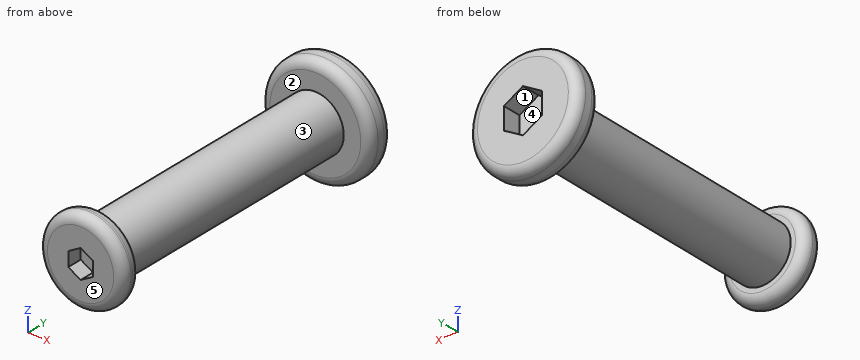
from build123d import *

# Parameters (mm, degrees)
SKETCH_1_R          = 2.9
EXTRUDE_1_DEPTH     = 1.4
CUT_EXTRUDE_1_DEPTH = 1
SKETCH_3_R          = 1.5
EXTRUDE_2_DEPTH     = 14
SKETCH_4_R          = 2.25
EXTRUDE_3_DEPTH     = 1.1
CUT_EXTRUDE_2_DEPTH = 0.8
FILLET_1_R          = 0.5


with BuildPart() as part:
    # 草图1 → 凸台-拉伸1 (new body)
    with BuildSketch(Plane(origin=(0, 0, 0), x_dir=(1, 0, 0), z_dir=(0, 1, 0))):
        with Locations(Location((0, 0, 0), (0, 0, 270))):
            Circle(SKETCH_1_R)
    extrude(amount=EXTRUDE_1_DEPTH)

    # 草图2 → 切除-拉伸1 (cut)
    with BuildSketch(Plane(origin=(0, 1.4, 0), x_dir=(1, 0, 0), z_dir=(0, 1, 0))):
        Polygon((1, 0.577350269), (0, 1.154700538), (-1, 0.577350269), (-1, -0.577350269), (0, -1.154700538), (1, -0.577350269), align=None)
    extrude(amount=-CUT_EXTRUDE_1_DEPTH, mode=Mode.SUBTRACT)

    # 草图3 → 凸台-拉伸2 (add)
    with BuildSketch(Plane.XZ):
        with Locations(Location((0, 0, 0), (0, 0, 270))):
            Circle(SKETCH_3_R)
    extrude(amount=EXTRUDE_2_DEPTH)

    # 草图4 → 凸台-拉伸3 (add)
    with BuildSketch(Plane.XZ.offset(14)):
        with Locations(Location((0, 0, 0), (0, 0, 270))):
            Circle(SKETCH_4_R)
    extrude(amount=EXTRUDE_3_DEPTH)

    # 草图5 → 切除-拉伸2 (cut)
    with BuildSketch(Plane.XZ.offset(15.1)):
        Polygon((0.65, 0.375277675), (0, 0.75055535), (-0.65, 0.375277675), (-0.65, -0.375277675), (0, -0.75055535), (0.65, -0.375277675), align=None)
    extrude(amount=-CUT_EXTRUDE_2_DEPTH, mode=Mode.SUBTRACT)

    # 圆角1
    fillet_1_edges = [part.edges().sort_by_distance(p)[0] for p in [
        (0, 0, -2.9),
        (0, -14, 2.25),
        (0, -15.1, 2.25),
        (0, 1.4, -2.9),
    ]]
    fillet(fillet_1_edges, radius=FILLET_1_R)


solid = part.part
Could you check a few things on this model? Use its own coordinates, in mm. Face numbers are marked on the shaded views. A direction names the side the tool comes from. Round coordinates to 2 decimals unless told otherwise and drop trailing zeros. Order: outer loops, then holes, each group sorted by start corner. A loop starts at its lowest first (then second) coordinate and runs counter-clockwise, first axis right, second up.
Q1. Imagine slicing it at B-B, the plane y = -3.25. List the corners of the cut face in (x, z) for me.
Geometry says:
outline: circle Ø3 at (0, 0)
Q2. I'm going to push flat-ended pins straight in: P1, Ø0.8, axis at y = -15, z = 0, coming from the +X side; P2, Ø0.7, axis at x = 0, z = 0, coming from the -Y side; P3, Ø1.5, axis at y = -8.5, z = 0, coming from the +X side. Where does each tip first touch, or does it pass through?
Geometry says:
P1: stops at x = 2.25
P2: stops at y = -14.3
P3: stops at x = 1.5
Q3. Which directions (+Z, -Z, +X, -X, +Y, -Y) give clear straight access to the entire face, cutting with the end or side of a thin tool? Please do the marked faces 4 and 5.
Geometry says:
face 4: +Y
face 5: +Z, -Z, +X, -X, -Y
Q4. Imagine slicing it at A-A, the plane z = 0. List the corners of the cut face in (x, y) for me, then the cut area to 3 significant figures.
Geometry says:
outline: (-2.9, 0.5) arc R0.5 ccw to (-2.4, 0) - (-1.5, 0) - (-1.5, -14) - (-1.75, -14) arc R0.5 ccw to (-2.25, -14.5) - (-2.25, -14.6) arc R0.5 ccw to (-1.75, -15.1) - (-0.65, -15.1) - (-0.65, -14.3) - (0.65, -14.3) - (0.65, -15.1) - (1.75, -15.1) arc R0.5 ccw to (2.25, -14.6) - (2.25, -14.5) arc R0.5 ccw to (1.75, -14) - (1.5, -14) - (1.5, 0) - (2.4, 0) arc R0.5 ccw to (2.9, 0.5) - (2.9, 0.9) arc R0.5 ccw to (2.4, 1.4) - (1, 1.4) - (1, 0.4) - (-1, 0.4) - (-1, 1.4) - (-2.4, 1.4) arc R0.5 ccw to (-2.9, 0.9) - close
area: 51.6 mm2
Q5. Please list where these lines run through material, in increasing order: probe 1 along Y at (x, z) = (0.2, 0.4); probe 2 along Y at (x, z) = (1.5, -1.3); probe 3 along Y at (x, z) = (-1.4, -1.1).
Geometry says:
probe 1: y = -14.3 to 0.4
probe 2: y = -15.04 to -14.06, 0 to 1.4
probe 3: y = -15.1 to -14, 0 to 1.4
Q6. Thinking about a two-plate mould opening in X: for the marked faces 1, 2 and 3, which applies, released by +X, released by -X, zero draft, split by the parting line, or undercut?
Geometry says:
face 1: undercut
face 2: zero draft
face 3: split by the parting line
